Design review of the part built by this model. Coordinates are the model's own, in mm. A direction names the side the tool comes from. Give positions to 0.01 mm unless a question says otherwise; leave off trailing zeros. Loops run counter-clockwise (first coordinate to the right, second up) from the corner with the lowest first, then second, coordinate; pieces in that order, holes last. Notation, with made-up numbers: (-27, -14) -> (2, -14) arc R25 cw to (2, 17) -> close; hole circle Ø1 at (21, -26). An arc over 180 degrees is marked (long way). Answer as CSV lines item,"result".
Autodesk Inventor part; units mm, degrees
ref_plane "YZ Plane" through (0, 0, 0) normal (1, 0, 0) x (0, 1, 0)
ref_plane "XZ Plane" through (0, 0, 0) normal (0, 1, 0) x (-1, 0, 0)
ref_plane "XY Plane" through (0, 0, 0) normal (0, 0, 1) x (1, 0, 0)
sketch "Boceto1" plane through (0, 0, 0) normal (0, 0, 1) x (1, 0, 0)
  line L0 (0, 0) -> (100, 0)
  line L1 (100, 0) -> (100, 500)
  line L2 (0, 500) -> (0, 0)
  line L3 (0, 500) -> (17.6777, 482.3223)
  line L4 (100, 500) -> (82.3223, 482.3223)
  line L5 (17.6777, 482.3223) -> (82.3223, 482.3223)
  line L6 (50, -100) -> (-150, -100)
revolve "Revolución1" add sketch "Boceto1" angle 360 about axis through (50, -100, 0) along (-1, 0, 0)
sketch "Boceto2" plane through (100, -100, 0) normal (1, 0, 0) x (0, 0, -1)
  circle A0 centre (0, 0) radius 600 construction
  circle A1 centre (-387.4756, 0) radius 35
  circle A2 centre (0, 0) radius 100 construction
  circle A3 centre (0, -387.4756) radius 35
  circle A4 centre (387.4756, 0) radius 35
  circle A5 centre (0, 387.4756) radius 35
  point P0 (0, 100)
  dimension "d13" = 360
extrude "Extrusión1" cut sketch "Boceto2" against normal through all
thicken "Engrosado1" operation add thickness 10 both sides no extend neighbours no toward (1, 0, 0) faces at (100, -375.8968, 274.6836)
thicken "Engrosado2" operation add thickness 10 both sides no extend neighbours no toward (-1, 0, 0) faces at (0, -375.8968, 274.6836)
sketch "Boceto3" plane through (110, -100, 0) normal (1, 0, 0) x (0, 0, -1)
  line L0 (25, 96.8246) -> (25, 125)
  line L1 (25, 125) -> (-25, 125)
  line L2 (-25, 125) -> (-25, 96.8246)
  line L3 (0, 100) -> (25, 125) construction
  line L4 (0, 100) -> (-25, 125) construction
  arc A0 (25, 96.8246) -> (-25, 96.8246) centre (0, 0) ccw
  point P0 (0, 100)
extrude "Extrusión2" cut sketch "Boceto3" against normal blind 120
sketch "Boceto4" plane through (110, -100, 0) normal (1, 0, 0) x (0, 0, -1)
  point P0 (0, 100)
properties part number "Polea_EjercicioClase"
Q1. We need section C-C, the plane x = 52. State the section outline as (y, z) points.
Filled sheet:
outline,"circle Ø1164.64 at (-100, 0); hole circle Ø70 at (-487.48, 0); hole circle Ø70 at (-100, -387.48); hole circle Ø70 at (-100, 387.48); hole (-3.18, -25) -> (25, -25) -> (25, 25) -> (-3.18, 25) arc R100 ccw (long way) to start; hole circle Ø70 at (287.48, 0)"
Q2. To check wall thickness, follow probe 1 along Y at (x, z) = (29, 0); probe 2 along Z at (x, y) = (1.5, -109); probe 3 along Y at (x, z) = (60, 19.5). State the ranges of each line that lie inside material, in increasing order. Write a range as from..to.
Filled sheet:
probe 1,"y = -682.32..-522.48, -452.48..-200, 25..252.48, 322.48..482.32"
probe 2,"z = -598.43..-421.3, -353.65..-99.59, 99.59..353.65, 421.3..598.43"
probe 3,"y = -682..-516.54, -458.41..-198.08, 25..258.41, 316.54..482"
Q3. Clearance check with flat-ended pins moving along their axes: pin 1 Ø2 at (x, z) = (94, -385) entering from +Y; pin 2 Ø6 at (x, z) = (18, 371) entering from -Y; pin 3 Ø5 at (x, y) = (29, -541) entering from -Z. State where each tip first meets the part, or that it passes through.
Filled sheet:
pin 1,"stops at y = 353.9"
pin 2,"stops at y = -553.02"
pin 3,"stops at z = -383.17"
Q4. We need section A-A, the plane z = 0. State the section outline as (x, y) points, and give its area (3 significant figures).
Filled sheet:
outline,"(-10, -700) -> (0, -700) -> (17.68, -682.32) -> (82.32, -682.32) -> (100, -700) -> (110, -700) -> (110, -522.48) -> (-10, -522.48) -> close; (-10, -452.48) -> (110, -452.48) -> (110, -200) -> (-10, -200) -> close; (-10, 25) -> (110, 25) -> (110, 252.48) -> (-10, 252.48) -> close; (-10, 322.48) -> (110, 322.48) -> (110, 500) -> (100, 500) -> (82.32, 482.32) -> (17.68, 482.32) -> (0, 500) -> (-10, 500) -> close"
area,"97,300 mm^2"
Q5. For faces 5 (the conical face through (16.572, -226.476, 569.554)), 6 (the flat face through (-10, -108, 125)), 7 (the flat face through (51, 11, -25)), list the 3-axis set-ups (+Z, -Z, +X, -X, +Y, -Y) from which the entire face can be reached by the end or side of a thin tool; tool diameter is ignored.
Filled sheet:
face 5,"none"
face 6,"+Z, -Z, -X, +Y, -Y"
face 7,"+X, -X"
Q6. We need section B-B, the plane y = -100. State the section outline as (x, z) points, and give its area (3 significant figures).
Filled sheet:
outline,"(-10, -600) -> (0, -600) -> (17.68, -582.32) -> (82.32, -582.32) -> (100, -600) -> (110, -600) -> (110, -422.48) -> (-10, -422.48) -> close; (-10, -352.48) -> (110, -352.48) -> (110, -100) -> (-10, -100) -> close; (-10, 100) -> (110, 100) -> (110, 352.48) -> (-10, 352.48) -> close; (-10, 422.48) -> (110, 422.48) -> (110, 600) -> (100, 600) -> (82.32, 582.32) -> (17.68, 582.32) -> (0, 600) -> (-10, 600) -> close"
area,"100,000 mm^2"
Q7. The part is to be moulded in two halves that separate along X. For faces 1 (the conical face through (83.428, -226.476, -569.554)), 2 (the flat face through (110, -108, 125)), 3 (the cylindrical face through (50.453, -226.236, -568.475)), 4 (the cylindrical face through (104.93, -542.225, -405.509)), say which applies: pulls with the +X half, pulls with the -X half, needs draft (parallel to the pull), parting line crosses it, or undercut.
Filled sheet:
face 1,"undercut"
face 2,"pulls with the +X half"
face 3,"undercut"
face 4,"needs draft"
